Geometry: final body of the model. Coordinates: model frame, mm. A direction names the side the tool comes from. Round coordinates to 2 decimals unless told otherwise and drop trailing zeros. Loops run counter-clockwise (first coordinate to the right, second up) from the corner with the lowest first, then second, coordinate; pieces in that order, holes last. Notation, with made-up numbers: M -2.5,-30 L 20.5,-30 A21 ccw 20.5,-12 Z; hole C 23.5,-38 d8. An arc over 180 degrees is marked long. Answer as a JSON object with one key per item and string values.
```python
from build123d import *

# Parameters (mm, degrees)
EXTRUDE_1_DEPTH     = 2
CUT_EXTRUDE_1_DEPTH = 10


with BuildPart() as part:
    # 스케치1 → 보스-돌출1 (new body)
    with BuildSketch(Plane.XY):
        Polygon((3, 16), (0, 13), (0, 3), (3, 0), (47, 0), (50, 3), (50, 13), (47, 16), align=None)
    extrude(amount=EXTRUDE_1_DEPTH)

    # 스케치2 → 컷-돌출1 (cut)
    with BuildSketch(Plane.XY.offset(2)):
        Polygon((46, 12.618802154), (42, 10.309401077), (42, 5.690598923), (46, 3.381197846), (50, 5.690598923), (50, 10.309401077), align=None)
    extrude(amount=-CUT_EXTRUDE_1_DEPTH, mode=Mode.SUBTRACT)


solid = part.part
```
1) First-contact query: pin 1 (1 mm diameter, centred on y = 7.5, z = 1, fed in from +X). Flat tip, straight axial feed; report the tip coordinate or a pass-through.
Geometry results:
{"pin 1": "x = 42"}
2) Set-up query: faces 5 (the face through (42, 8, 1)), 6 (the face through (1, 2, 1)), 7 (the face through (47.97, 4.52, 1.01)). Return all of +Z, -Z, +X, -X, +Y, -Y with unobstructed straight access to the full face (end or side cutting, diameter ignored); none if empty.
Geometry results:
{"face 5": "+Z, -Z, +X", "face 6": "+Z, -Z, -X, -Y", "face 7": "+Z, -Z"}
3) Pull-direction query (X, two-part tool) for faces 1 (the face through (25, 16, 1)), 2 (the face through (50, 12, 1)), 3 (the face through (48.028, 11.448, 1.014)), 4 (the face through (43.972, 4.552, 1.014)); classes: +X half, -X half, draft (parallel to the pull), parting line (faces both ways), or undercut.
Geometry results:
{"face 1": "draft", "face 2": "+X half", "face 3": "undercut", "face 4": "undercut"}
4) Line query: probe 1 along X at (y, z) = (6.75, 0.8); probe 2 along X at (y, z) = (12.5, 1.3); probe 3 along Y at (x, z) = (47.5, 1.15). Output: solid intervals per line, ascending.
Geometry results:
{"probe 1": "0 to 42", "probe 2": "0 to 45.79, 46.21 to 50", "probe 3": "0.5 to 4.25, 11.75 to 15.5"}
5) Cut plane D-D on y = 9.25. Return the cut outline in (x, z).
Geometry results:
{"outline": "M 0,0 L 42,0 L 42,2 L 0,2 Z"}
6) Cut plane A-A on z = 0.95. Return the cut outline in (x, y), and give its area (3 significant figures).
Geometry results:
{"outline": "M 0,3 L 3,0 L 47,0 L 50,3 L 50,5.69 L 46,3.38 L 42,5.69 L 42,10.31 L 46,12.62 L 50,10.31 L 50,13 L 47,16 L 3,16 L 0,13 Z", "area": "727 mm2"}
7) Cut plane B-B on y = 11.5. Return the cut outline in (x, z).
Geometry results:
{"outline": "M 0,0 L 44.06,0 L 44.06,2 L 0,2 Z; M 47.94,0 L 50,0 L 50,2 L 47.94,2 Z"}
8) Cut plane C-C on y = 2. Return the cut outline in (x, z), and give its area (3 significant figures).
Geometry results:
{"outline": "M 1,0 L 49,0 L 49,2 L 1,2 Z", "area": "96.0 mm2"}
